from build123d import *

# Parameters (mm, degrees)
SKETCH1_R               = 2.286
BOSS_EXTRUDE1_DEPTH     = 35.814
SKETCH3_W               = 13.716
SKETCH3_H               = 60.96
CUT_EXTRUDE2_DEPTH      = 34.544
SKETCH4_W               = 3.81
SKETCH4_H               = 6.35
CUT_EXTRUDE3_DEPTH      = 114.792
SKETCH5_W               = 97.536
SKETCH5_H               = 2.032
CUT_EXTRUDE6_DEPTH      = 3.048
LPATTERN1_COUNT         = 9
LPATTERN1_PITCH         = 3.175
MIRROR1_COPY_1_SKETCH_W = 97.536
MIRROR1_COPY_1_SKETCH_H = 2.032
MIRROR1_COPY_1_DEPTH    = 3.048
MIRROR1_COPY_2_SKETCH_W = 97.536
MIRROR1_COPY_2_SKETCH_H = 2.032
MIRROR1_COPY_2_DEPTH    = 3.048
MIRROR1_COPY_3_SKETCH_W = 97.536
MIRROR1_COPY_3_SKETCH_H = 2.032
MIRROR1_COPY_3_DEPTH    = 3.048
MIRROR1_COPY_4_SKETCH_W = 97.536
MIRROR1_COPY_4_SKETCH_H = 2.032
MIRROR1_COPY_4_DEPTH    = 3.048
MIRROR1_COPY_5_SKETCH_W = 97.536
MIRROR1_COPY_5_SKETCH_H = 2.032
MIRROR1_COPY_5_DEPTH    = 3.048
MIRROR1_COPY_6_SKETCH_W = 97.536
MIRROR1_COPY_6_SKETCH_H = 2.032
MIRROR1_COPY_6_DEPTH    = 3.048


with BuildPart() as part:
    # Sketch1 → Boss-Extrude1 (new body)
    with BuildSketch(Plane(origin=(0, 0, 0), x_dir=(1, 0, 0), z_dir=(0, 1, 0))):
        with BuildLine():
            Line((0, 11.938), (0, 55.118))
            ThreePointArc((0, 55.118), (-2.603820715, 61.404179285), (-8.89, 64.008))
            Line((-8.89, 64.008), (-13.716, 64.008))
            Line((-13.716, 64.008), (-13.716, 66.04))
            Line((-13.716, 66.04), (-113.792, 66.04))
            Line((-113.792, 66.04), (-113.792, 64.008))
            Line((-113.792, 64.008), (-118.618, 64.008))
            ThreePointArc((-118.618, 64.008), (-124.904179285, 61.404179285), (-127.508, 55.118))
            Line((-127.508, 55.118), (-127.508, 11.938))
            ThreePointArc((-127.508, 11.938), (-124.904179285, 5.651820715), (-118.618, 3.048))
            Line((-118.618, 3.048), (-113.792, 3.048))
            Line((-113.792, 3.048), (-113.792, 1.016))
            Line((-113.792, 1.016), (-13.716, 1.016))
            Line((-13.716, 1.016), (-13.716, 3.048))
            Line((-13.716, 3.048), (-8.89, 3.048))
            ThreePointArc((-8.89, 3.048), (-2.603820715, 5.651820715), (0, 11.938))
        make_face()
        with Locations((-120.65, 33.528)):
            Circle(SKETCH1_R, mode=Mode.SUBTRACT)
        with Locations((-6.858, 33.528)):
            Circle(SKETCH1_R, mode=Mode.SUBTRACT)
        with BuildLine():
            Line((-118.367709413, 17.018), (-118.325280939, 12.192))
            ThreePointArc((-118.325280939, 12.192), (-120.65, 9.867280939), (-122.974719061, 12.192))
            Line((-122.974719061, 12.192), (-122.932290587, 17.018))
            ThreePointArc((-122.932290587, 17.018), (-120.65, 19.300290587), (-118.367709413, 17.018))
        make_face(mode=Mode.SUBTRACT)
        with BuildLine():
            Line((-122.974719061, 54.864), (-122.932290587, 50.038))
            ThreePointArc((-122.932290587, 50.038), (-120.65, 47.755709413), (-118.367709413, 50.038))
            Line((-118.367709413, 50.038), (-118.325280939, 54.864))
            ThreePointArc((-118.325280939, 54.864), (-120.65, 57.188719061), (-122.974719061, 54.864))
        make_face(mode=Mode.SUBTRACT)
        with BuildLine():
            Line((-9.140290587, 50.038), (-9.182719061, 54.864))
            ThreePointArc((-9.182719061, 54.864), (-6.858, 57.188719061), (-4.533280939, 54.864))
            Line((-4.533280939, 54.864), (-4.575709413, 50.038))
            ThreePointArc((-4.575709413, 50.038), (-6.858, 47.755709413), (-9.140290587, 50.038))
        make_face(mode=Mode.SUBTRACT)
        with BuildLine():
            Line((-4.533280939, 12.192), (-4.575709413, 17.018))
            ThreePointArc((-4.575709413, 17.018), (-6.858, 19.300290587), (-9.140290587, 17.018))
            Line((-9.140290587, 17.018), (-9.182719061, 12.192))
            ThreePointArc((-9.182719061, 12.192), (-6.858, 9.867280939), (-4.533280939, 12.192))
        make_face(mode=Mode.SUBTRACT)
    extrude(amount=BOSS_EXTRUDE1_DEPTH)

    # Sketch3 → Cut-Extrude2 (cut)
    with BuildSketch(Plane(origin=(0, 35.814, 0), x_dir=(1, 0, 0), z_dir=(0, 1, 0))):
        with Locations((-6.858, 33.528)):
            Rectangle(SKETCH3_W, SKETCH3_H)
        with Locations((-120.65, 33.528)):
            Rectangle(SKETCH3_W, SKETCH3_H)
    extrude(amount=-CUT_EXTRUDE2_DEPTH, mode=Mode.SUBTRACT)

    # Sketch4 → Cut-Extrude3 (cut, through all)
    with BuildSketch(Plane.ZY.offset(113.792)):
        Polygon((-17.78, 35.814), (-1.016, 33.274), (-1.016, 35.814), align=None)
        with Locations((-64.135, 19.431)):
            Rectangle(SKETCH4_W, SKETCH4_H)
        with Locations((-2.921, 19.431)):
            Rectangle(SKETCH4_W, SKETCH4_H)
        Polygon((-66.04, 33.274), (-66.04, 35.814), (-49.276, 35.814), align=None)
    extrude(amount=-CUT_EXTRUDE3_DEPTH, mode=Mode.SUBTRACT)

    # Sketch5 → Cut-Extrude6 (cut)
    with BuildSketch(Plane.XY.offset(-1.016)):
        with Locations((-63.754, 30.48)):
            Rectangle(SKETCH5_W, SKETCH5_H)
    cut_extrude6 = extrude(amount=-CUT_EXTRUDE6_DEPTH, mode=Mode.SUBTRACT)

    # LPattern1: Cut-Extrude6 ×9, 2 skipped
    with Locations(*[(0, -i * LPATTERN1_PITCH, 0) for i in range(1, LPATTERN1_COUNT) if i not in (3, 4)]):
        add(cut_extrude6, mode=Mode.SUBTRACT)

    # Mirror1: Cut-Extrude6 across plane
    add(cut_extrude6.mirror(Plane.XY.offset(-33.528)), mode=Mode.SUBTRACT)

    # Mirror1 copy 1 sketch → Mirror1 copy 1 (cut)
    with BuildSketch(Plane(origin=(0, -3.175, -66.04), x_dir=(1, 0, 0), z_dir=(0, 0, -1))):
        with Locations((-63.754, -30.48)):
            Rectangle(MIRROR1_COPY_1_SKETCH_W, MIRROR1_COPY_1_SKETCH_H)
    extrude(amount=-MIRROR1_COPY_1_DEPTH, mode=Mode.SUBTRACT)

    # Mirror1 copy 2 sketch → Mirror1 copy 2 (cut)
    with BuildSketch(Plane(origin=(0, -6.35, -66.04), x_dir=(1, 0, 0), z_dir=(0, 0, -1))):
        with Locations((-63.754, -30.48)):
            Rectangle(MIRROR1_COPY_2_SKETCH_W, MIRROR1_COPY_2_SKETCH_H)
    extrude(amount=-MIRROR1_COPY_2_DEPTH, mode=Mode.SUBTRACT)

    # Mirror1 copy 3 sketch → Mirror1 copy 3 (cut)
    with BuildSketch(Plane(origin=(0, -15.875, -66.04), x_dir=(1, 0, 0), z_dir=(0, 0, -1))):
        with Locations((-63.754, -30.48)):
            Rectangle(MIRROR1_COPY_3_SKETCH_W, MIRROR1_COPY_3_SKETCH_H)
    extrude(amount=-MIRROR1_COPY_3_DEPTH, mode=Mode.SUBTRACT)

    # Mirror1 copy 4 sketch → Mirror1 copy 4 (cut)
    with BuildSketch(Plane(origin=(0, -19.05, -66.04), x_dir=(1, 0, 0), z_dir=(0, 0, -1))):
        with Locations((-63.754, -30.48)):
            Rectangle(MIRROR1_COPY_4_SKETCH_W, MIRROR1_COPY_4_SKETCH_H)
    extrude(amount=-MIRROR1_COPY_4_DEPTH, mode=Mode.SUBTRACT)

    # Mirror1 copy 5 sketch → Mirror1 copy 5 (cut)
    with BuildSketch(Plane(origin=(0, -22.225, -66.04), x_dir=(1, 0, 0), z_dir=(0, 0, -1))):
        with Locations((-63.754, -30.48)):
            Rectangle(MIRROR1_COPY_5_SKETCH_W, MIRROR1_COPY_5_SKETCH_H)
    extrude(amount=-MIRROR1_COPY_5_DEPTH, mode=Mode.SUBTRACT)

    # Mirror1 copy 6 sketch → Mirror1 copy 6 (cut)
    with BuildSketch(Plane(origin=(0, -25.4, -66.04), x_dir=(1, 0, 0), z_dir=(0, 0, -1))):
        with Locations((-63.754, -30.48)):
            Rectangle(MIRROR1_COPY_6_SKETCH_W, MIRROR1_COPY_6_SKETCH_H)
    extrude(amount=-MIRROR1_COPY_6_DEPTH, mode=Mode.SUBTRACT)


solid = part.part
Can you work these out from the model? Positions are in its coordinate system, mm. A direction names the side the tool comes from. Give positions to 0.01 mm unless a question says otherwise; leave off trailing zeros. Loops run counter-clockwise (first coordinate to the right, second up) from the corner with the lowest first, then second, coordinate; pieces in that order, holes last. Notation, with made-up numbers: (59, -5.5) -> (93, -5.5) arc R13 ccw to (93, 11.5) -> close; hole circle Ø7 at (47, 89). An arc over 180 degrees is marked (long way). Return JSON: item names as keys, results as strings.
Q1. I want a section at A-A, the plane x = -120.65. List the corners of the cut face in (y, z) for me.
Checks:
{"outline": "(0, -63.77) -> (1.27, -63.77) -> (1.27, -57.19) -> (0, -57.19) -> close; (0, -47.76) -> (1.27, -47.76) -> (1.27, -35.81) -> (0, -35.81) -> close; (0, -31.24) -> (1.27, -31.24) -> (1.27, -19.3) -> (0, -19.3) -> close; (0, -9.87) -> (1.27, -9.87) -> (1.27, -3.28) -> (0, -3.28) -> close"}
Q2. I want a section at C-C, the plane y = 19.5. List the corners of the cut face in (x, z) for me.
Checks:
{"outline": "(-113.79, -62.23) -> (-13.72, -62.23) -> (-13.72, -4.83) -> (-113.79, -4.83) -> close"}
Q3. I want a section at B-B, the plane z = -29. List the corners of the cut face in (x, y) for me, then the cut area to 3 significant figures.
Checks:
{"outline": "(-127.51, 0) -> (0, 0) -> (0, 1.27) -> (-13.72, 1.27) -> (-13.72, 35.81) -> (-113.79, 35.81) -> (-113.79, 1.27) -> (-127.51, 1.27) -> close", "area": "3,620 mm2"}
Q4. On a 3-axis mill with a long thin cutter (end or side, diameter ignored), from which of +Z, -Z, +X, -X, +Y, -Y can I reach the whole of each face in a straight line? I mean faces 1 (the face through (-64, 26.289, -65)), 2 (the face through (-6.909, 0.626, -9.868)), 3 (the face through (-64, 9.271, -3)), 4 (the face through (-64, 19, -4.826)). Say none if no direction works.
Checks:
{"face 1": "-Z", "face 2": "+Y, -Y", "face 3": "+Z", "face 4": "+Z, +X, -X"}
Q5. For pin 1 Ø6 at (y, z) = (13.5, -29.5) entering from -X; pin 2 Ø0.6 at (x, y) = (-11.5, 0.5) entering from -Z; pin 3 Ø1.6 at (x, y) = (-86.5, 30.5) entering from +Z, each with a flat end and sliding along its axis, tell me the tip position at first contact or that it passes through.
Checks:
{"pin 1": "stops at x = -113.79", "pin 2": "stops at z = -64.01", "pin 3": "stops at z = -4.06"}
Q6. I want a section at D-D, the plane z = -8.5. List the corners of the cut face in (x, y) for me, then the cut area to 3 significant figures.
Checks:
{"outline": "(-126.82, 0) -> (-0.69, 0) -> (-0.69, 1.27) -> (-13.72, 1.27) -> (-13.72, 34.41) -> (-113.79, 34.41) -> (-113.79, 1.27) -> (-126.82, 1.27) -> close", "area": "3,480 mm2"}
Q7. We'd pull the mould along Y, two halves only. Please class faces 5 (the face through (-64, 10.414, -65)), 6 (the face through (-7.156, 0.626, -35.795)), 7 (the face through (-64.455, 34.562, -9.515)): released by +Y, released by -Y, zero draft, split by the parting line, or undercut.
Checks:
{"face 5": "undercut", "face 6": "zero draft", "face 7": "released by +Y"}
Q8. I need wall thicknesses on probe 1 along Z at (x, y) = (-120.65, 0.8); probe 2 along X at (y, z) = (30.5, -13.5); probe 3 along X at (y, z) = (30.5, -4). Which ranges of each line are inside material? Lowest first, please.
Checks:
{"probe 1": "z = -63.77 to -57.19, -47.76 to -35.81, -31.24 to -19.3, -9.87 to -3.28", "probe 2": "x = -113.79 to -13.72", "probe 3": "x = -113.79 to -112.52, -14.99 to -13.72"}
